Check sheet for the drawn part. Datum: minimum x, y, z corner. Units: mm. A direction names the side the tool comes from. Give positions to 0.01 mm unless a question says otherwise; leave off trailing zeros. Loops run counter-clockwise (first coordinate to the right, second up) from the corner with the lowest first, then second, coordinate; pieces in that order, holes last. Notation, with made-up numbers: M 68,82 L 126,82 A26 cw 126,112 Z; hole C -29,-14 d2. An arc over 180 degrees is marked long. Write each question's results on one line, items separated by ' | '. Start each with the question number.
1. Sectioned sample at B-B on z = 11.5. Record the cut outline in (x, y), and give its area (3 significant figures).
2. Sectioned sample at C-C on z = 26. Record the cut outline in (x, y), and give its area (3 significant figures).
3. Sectioned sample at D-D on y = 19.25. Record the cut outline in (x, z), and give its area (3 significant figures).
4. Material ranges on line 1 along X through (y, z) = (16, 11.5); line 2 along Y through (x, z) = (10.25, 15), recorded low to high.
5. Sectioned sample at A-A on y = 4.5. Record the cut outline in (x, z).
6. Tool access check on the marked faces 1, 2, 3, 4 and 5. Record the directions out of +Z, -Z, +X, -X, +Y, -Y that give a thin tool (end or side, any length) a straight path to the whole face; none if there is none.
7. Go/stop test with flat-tipped pins: pin 1 (4 mm diameter, centred on x = 16.5, y = 16.5, fed in from +Z); pin 2 (3 mm diameter, centred on x = 10, y = 14.5, fed in from +Z); pin 3 (4 mm diameter, centred on x = 17.5, y = 8.5, fed in from +Z); pin 4 (5 mm diameter, centred on y = 20, z = 6, fed in from -X). Record where each tip stops, or that it passes through.
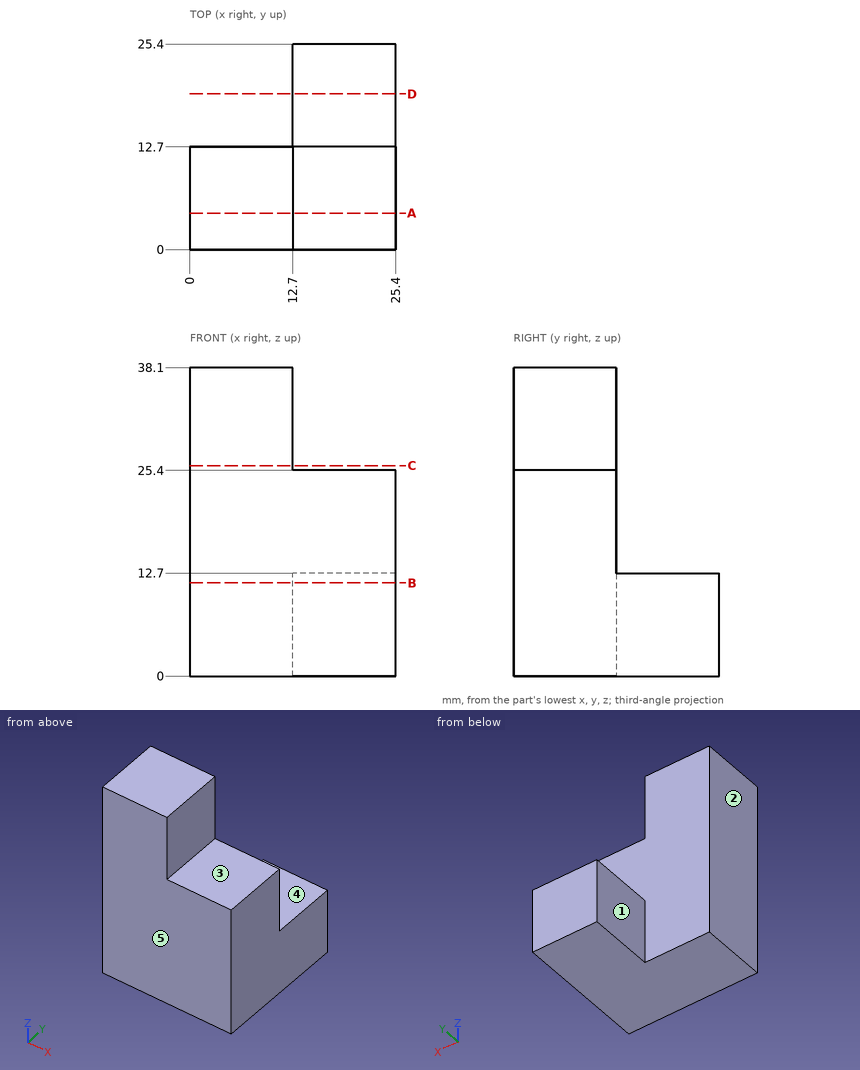
Output values:
1) outline: M 0,0 L 25.4,0 L 25.4,25.4 L 12.7,25.4 L 12.7,12.7 L 0,12.7 Z | area: 484 mm2
2) outline: M 0,0 L 12.7,0 L 12.7,12.7 L 0,12.7 Z | area: 161 mm2
3) outline: M 12.7,0 L 25.4,0 L 25.4,12.7 L 12.7,12.7 Z | area: 161 mm2
4) line 1: 12.7 to 25.4 | line 2: 0 to 12.7
5) outline: M 0,0 L 25.4,0 L 25.4,25.4 L 12.7,25.4 L 12.7,38.1 L 0,38.1 Z
6) face 1: +Z, -Z, -X, +Y | face 2: +Z, -Z, -X, +Y, -Y | face 3: +Z, +X, +Y, -Y | face 4: +Z, +X, -X, +Y | face 5: +Z, -Z, +X, -X, -Y
7) pin 1: z = 12.7 | pin 2: through | pin 3: z = 25.4 | pin 4: x = 12.7
